from build123d import *

# Parameters (mm, degrees)
F0_R     = 5.117058
F0_R_2   = 18.848799
F0_R_3   = 9.024126
F1_DEPTH = 30
F6_DEPTH = 10.785379
F2_R     = 20.800257
F2_R_2   = 29.342009
F2_R_3   = 9.581233
F3_DEPTH = 17.246447
F4_DEPTH = 0.934202


with BuildPart() as f1:
    # F0 (on Front) → F1 (new body)
    with BuildSketch(Plane.XZ):
        with BuildLine():
            ThreePointArc((8.222921, 28.166239), (23.475844, 17.602222), (29.342009, 0))
            ThreePointArc((29.342009, 0), (23.475844, -17.602222), (8.222921, -28.166239))
            Line((8.222921, -28.166239), (73.19784, -9.197302))
            ThreePointArc((73.19784, -9.197302), (60.931524, 0), (73.19784, 9.197302))
            Line((73.19784, 9.197302), (8.222921, 28.166239))
        make_face()
        with BuildLine():
            ThreePointArc((80.09399, 0), (78.178474, 5.747766), (73.19784, 9.197302))
            ThreePointArc((73.19784, 9.197302), (60.931524, 0), (73.19784, -9.197302))
            ThreePointArc((73.19784, -9.197302), (78.178474, -5.747766), (80.09399, 0))
        make_face()
        with Locations((70.512757, 0)):
            Circle(F0_R, mode=Mode.SUBTRACT)
        with Locations((70.512757, 0)):
            Circle(F0_R)
        with BuildLine():
            ThreePointArc((8.222921, -28.166239), (23.475844, -17.602222), (29.342009, 0))
            ThreePointArc((29.342009, 0), (23.475844, 17.602222), (8.222921, 28.166239))
            ThreePointArc((8.222921, 28.166239), (2.321575, 29.250022), (-3.676847, 29.110724))
            ThreePointArc((-3.676847, 29.110724), (-29.342009, 0), (-3.676847, -29.110724))
            ThreePointArc((-3.676847, -29.110724), (2.321575, -29.250022), (8.222921, -28.166239))
        make_face()
        Circle(F0_R_2, mode=Mode.SUBTRACT)
        Circle(F0_R_2)
        with BuildLine():
            ThreePointArc((-3.676847, -29.110724), (-29.342009, 0), (-3.676847, 29.110724))
            Line((-3.676847, 29.110724), (-70.771454, 20.636302))
            ThreePointArc((-70.771454, 20.636302), (-54.409335, 15.602342), (-47.364717, 0))
            ThreePointArc((-47.364717, 0), (-54.409335, -15.602342), (-70.771454, -20.636302))
            Line((-70.771454, -20.636302), (-3.676847, -29.110724))
        make_face()
        with BuildLine():
            ThreePointArc((-47.364717, 0), (-54.409335, 15.602342), (-70.771454, 20.636302))
            ThreePointArc((-70.771454, 20.636302), (-88.965232, 0), (-70.771454, -20.636302))
            ThreePointArc((-70.771454, -20.636302), (-54.409335, -15.602342), (-47.364717, 0))
        make_face()
        with Locations((-68.164974, 0)):
            Circle(F0_R_3, mode=Mode.SUBTRACT)
        with Locations((-68.164974, 0)):
            Circle(F0_R_3)
    extrude(amount=F1_DEPTH)

    # F0 (on Front) → F6 (cut)
    with BuildSketch(Plane.XZ):
        with Locations((-68.164974, 0)):
            Circle(F0_R_3)
        Circle(F0_R_2)
        with Locations((70.512757, 0)):
            Circle(F0_R)
    extrude(amount=F6_DEPTH, mode=Mode.SUBTRACT)

    # F2 (on offset) → F3 (join)
    with BuildSketch(Plane.XZ.offset(30)):
        with Locations((-68.947569, 0)):
            Circle(F2_R)
        with Locations((-0.782594, 0)):
            Circle(F2_R_2)
        with Locations((69.730163, 0)):
            Circle(F2_R_3)
    extrude(amount=-F3_DEPTH)

    # F0 (on Front) → F4 (cut)
    with BuildSketch(Plane.XZ):
        with BuildLine():
            ThreePointArc((-47.364717, 0), (-54.409335, 15.602342), (-70.771454, 20.636302))
            ThreePointArc((-70.771454, 20.636302), (-88.965232, 0), (-70.771454, -20.636302))
            ThreePointArc((-70.771454, -20.636302), (-54.409335, -15.602342), (-47.364717, 0))
        make_face()
        with Locations((-68.164974, 0)):
            Circle(F0_R_3, mode=Mode.SUBTRACT)
        with BuildLine():
            ThreePointArc((8.222921, -28.166239), (23.475844, -17.602222), (29.342009, 0))
            ThreePointArc((29.342009, 0), (23.475844, 17.602222), (8.222921, 28.166239))
            ThreePointArc((8.222921, 28.166239), (2.321575, 29.250022), (-3.676847, 29.110724))
            ThreePointArc((-3.676847, 29.110724), (-29.342009, 0), (-3.676847, -29.110724))
            ThreePointArc((-3.676847, -29.110724), (2.321575, -29.250022), (8.222921, -28.166239))
        make_face()
        Circle(F0_R_2, mode=Mode.SUBTRACT)
        with BuildLine():
            ThreePointArc((80.09399, 0), (78.178474, 5.747766), (73.19784, 9.197302))
            ThreePointArc((73.19784, 9.197302), (60.931524, 0), (73.19784, -9.197302))
            ThreePointArc((73.19784, -9.197302), (78.178474, -5.747766), (80.09399, 0))
        make_face()
        with Locations((70.512757, 0)):
            Circle(F0_R, mode=Mode.SUBTRACT)
    extrude(amount=-F4_DEPTH, mode=Mode.SUBTRACT)


solid = f1.part
Design review of the part built by this model. Coordinates are the model's own, in mm. A direction names the side the tool comes from. Coordinates: 2 decimals unless noted, no trailing zeros. Loops run counter-clockwise (first coordinate to the right, second up) from the corner with the lowest first, then second, coordinate; pieces in that order, holes last. Notation, with made-up numbers: (53, 61) - (64, 61) arc R26 cw to (64, 89) - close; hole circle Ø1 at (14.5, 7.5). An arc over 180 degrees is marked (long way). Use CSV: the item, a comma, the result in double quotes. Start each with the question number.
1. For faces 1 (the cylindrical face through (-88.96, -6.29, 0.42)), 2 (the cylindrical face through (-14.958, -5.317, -11.469)), 3 (the flat face through (-36.754, -14.79, 24.933)), list the 3-axis set-ups (+Z, -Z, +X, -X, +Y, -Y) from which the entire face can be reached by the end or side of a thin tool; tool diameter is ignored.
2. Add section B-B on z = 1.5. Give the boundary of the cut face in (x, y), plus the area to 3 significant figures.
3. Add section A-A on y = -5.5. Give the boundary of the cut face in (x, z), plus the area to 3 significant figures.
4. Add section D-D on y = -15.75. Give the boundary of the cut face in (x, z), plus the area to 3 significant figures.
5. Add section C-C on x = 12. Give the boundary of the cut face in (y, z).
6. Clearance check with flat-ended pins moving along their axes: pin 1 (2 mm diameter, centred on y = -12.5, z = -18, fed in from -X); pin 2 (2 mm diameter, centred on x = 1.5, y = -15, fed in from +Z); pin 3 (1.5 mm diameter, centred on x = 32, y = -14.5, fed in from -Z); pin 4 (0.5 mm diameter, centred on x = -5, z = -29, fed in from +Y). State where each tip first meets the part, or that it passes through.
7. To check wall thickness, follow probe 1 along Z at (x, y) = (0, -4.5); probe 2 along X at (y, z) = (-5, 8); probe 3 along X at (y, z) = (-9.25, 4). State the ranges of each line that lie inside material, in increasing order.
8. Mouldability with a two-part tool opening along Z and no side actions: class faces 4 (the flat face through (0, -10.785, 0)), 5 (the flat face through (70, -10.785, 0)), 6 (the flat face through (-6, -30, 0)), 7 (the cylindrical face through (-3.67, -21.5, -29.2)) as released by +Z, released by -Z, zero draft, split by the parting line, or undercut.
Resolved:
1,face 1,"-X, +Y"
1,face 2,"+Y"
1,face 3,"+Z, -X, +Y, -Y"
2,outline,"(-89.69, -30) - (79.98, -30) - (79.98, 0) - (75.41, 0) - (75.41, -10.79) - (65.62, -10.79) - (65.62, 0) - (18.79, 0) - (18.79, -10.79) - (-18.79, -10.79) - (-18.79, 0) - (-59.27, 0) - (-59.27, -10.79) - (-77.06, -10.79) - (-77.06, 0) - (-88.91, 0) - (-88.91, -12.75) - (-89.69, -12.75) - close"
2,area,"4,380 mm2"
3,outline,"(-70.77, -20.64) - (-3.68, -29.11) arc R29.34 ccw to (8.22, -28.17) - (73.2, -9.2) arc R9.58 ccw to (73.2, 9.2) - (8.22, 28.17) arc R29.34 ccw to (-3.68, 29.11) - (-70.77, 20.64) arc R20.8 ccw to start; hole circle Ø18.05 at (-68.16, 0); hole circle Ø37.7 at (0, 0); hole circle Ø10.23 at (70.51, 0)"
3,area,"5,670 mm2"
4,outline,"(-69.54, -20.79) - (-6.83, -28.71) arc R29.34 ccw to (-0.39, -29.34) arc R29.34 ccw to (8.22, -28.17) - (73.2, -9.2) arc R9.58 ccw to (73.2, 9.2) - (8.22, 28.17) arc R29.34 ccw to (-0.39, 29.34) arc R29.34 ccw to (-6.83, 28.71) - (-69.54, 20.79) arc R20.8 ccw to start"
4,area,"7,150 mm2"
5,outline,"(-30, -27.06) - (0, -27.06) - (0, -14.54) - (-10.79, -14.54) - (-10.79, 14.54) - (0, 14.54) - (0, 27.06) - (-30, 27.06) - close"
6,pin 1,"x = -80.89"
6,pin 2,"z = 29.34"
6,pin 3,"z = -21.44"
6,pin 4,"y = 0"
7,probe 1,"-29.34 to -18.85, 18.85 to 29.34"
7,probe 2,"-87.37 to -72.34, -63.99 to -17.07, 17.07 to 75.79"
7,probe 3,"-88.58 to -76.25, -60.08 to -18.42, 18.42 to 67.32, 73.7 to 79.22"
8,face 4,"undercut"
8,face 5,"undercut"
8,face 6,"zero draft"
8,face 7,"released by -Z"
